For this review, take the finished solid that the model builds, in its own axes (mm). Face numbers are marked on the shaded views. A direction names the side the tool comes from. Coordinates: 2 decimals unless noted, no trailing zeros. Write each loop counter-clockwise with the first axis right and the second up, starting at its lowest first coordinate (ties: lowest second). Pieces come first, ordered by that corner, then holes. Notation, with made-up numbers: M 14,-18 L 48,-18 A11 ccw 48,3 Z; hole C 32.25,87 d7. An arc over 180 degrees is marked long. Return JSON: item names as keys, results as strings.
```python
from build123d import *

# Parameters (mm, degrees)
F0_R     = 3.8651
F1_DEPTH = 5.41
F2_R     = 2.977189
F2_R_2   = 1.369861
F3_DEPTH = 2
F4_DEPTH = 1


with BuildPart() as f1:
    # F0 (on Front) → F1 (new body)
    with BuildSketch(Plane.XZ):
        with Locations((30.719768, 18.937557)):
            Circle(F0_R)
        with BuildLine():
            ThreePointArc((28.998524, 19.481013), (29.488314, 20.257233), (30.296515, 20.692231))
            Line((30.296515, 20.692231), (30.296515, 21.202457))
            Line((30.296515, 21.202457), (31.296515, 21.202457))
            Line((31.296515, 21.202457), (31.296515, 20.647933))
            ThreePointArc((31.296515, 20.647933), (32.008417, 20.201443), (32.441011, 19.481013))
            Line((32.441011, 19.481013), (32.984868, 19.481013))
            Line((32.984868, 19.481013), (32.984868, 18.481013))
            Line((32.984868, 18.481013), (32.466076, 18.481013))
            ThreePointArc((32.466076, 18.481013), (32.039681, 17.706356), (31.296515, 17.22718))
            Line((31.296515, 17.22718), (31.296515, 16.672457))
            Line((31.296515, 16.672457), (30.296515, 16.672457))
            Line((30.296515, 16.672457), (30.296515, 17.182882))
            ThreePointArc((30.296515, 17.182882), (29.455634, 17.64915), (28.973459, 18.481013))
            Line((28.973459, 18.481013), (28.454868, 18.481013))
            Line((28.454868, 18.481013), (28.454868, 19.481013))
            Line((28.454868, 19.481013), (28.998524, 19.481013))
        make_face(mode=Mode.SUBTRACT)
    extrude(amount=F1_DEPTH)

    # F2 (on Front) → F3 (join)
    with BuildSketch(Plane.XZ):
        with Locations((30.680057, 18.935421)):
            Circle(F2_R)
        with Locations((30.680057, 18.935421)):
            Circle(F2_R_2, mode=Mode.SUBTRACT)
    extrude(amount=F3_DEPTH)

    # F2 (on Front) → F4 (cut)
    with BuildSketch(Plane.XZ):
        with Locations((30.680057, 18.935421)):
            Circle(F2_R)
        with Locations((30.680057, 18.935421)):
            Circle(F2_R_2, mode=Mode.SUBTRACT)
    extrude(amount=F4_DEPTH, mode=Mode.SUBTRACT)


solid = f1.part
```
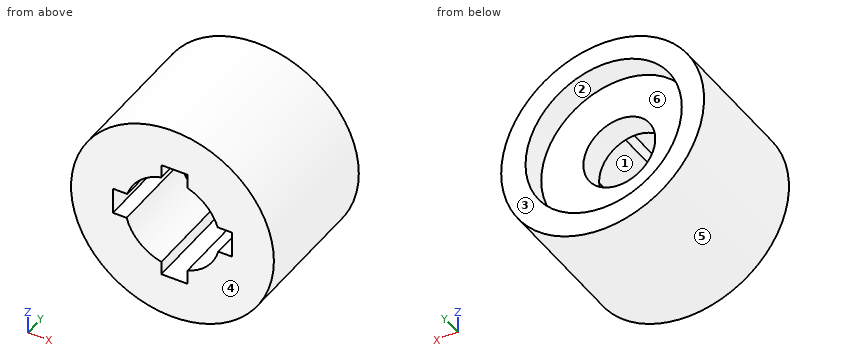
1. We need section A-A (z = 18.75). State the section outline as (x, y) points.
Checks:
{"outline": "M 26.86,-5.41 L 28.45,-5.41 L 28.45,-2 L 29.32,-2 L 29.32,-1 L 27.71,-1 L 27.71,0 L 26.86,0 Z; M 32.04,-2 L 32.98,-2 L 32.98,-5.41 L 34.58,-5.41 L 34.58,0 L 33.65,0 L 33.65,-1 L 32.04,-1 Z"}
2. Wall thickness on L1, parallel to Y at x = 29.5, z = 18; L2, parallel to Z at x = 32.5, y = -2.35; L3, parallel to Z at x = 29.75, y = -3: over which ranges is each line inside the solid? List them lowest first. Write a range as from..to.
Checks:
{"L1": "-2..-1", "L2": "15.51..18.48, 19.48..22.37", "L3": "15.2..17.42, 20.46..22.68"}
3. We need section B-B (y = -4.1). State the section outline as (x, z) points (3 decimals), plus the area to 3 significant figures.
Checks:
{"outline": "C 30.72,18.938 d7.73; hole M 28.455,18.481 L 28.973,18.481 A1.805 ccw 30.297,17.183 L 30.297,16.672 L 31.297,16.672 L 31.297,17.227 A1.805 ccw 32.466,18.481 L 32.985,18.481 L 32.985,19.481 L 32.441,19.481 A1.805 ccw 31.297,20.648 L 31.297,21.202 L 30.297,21.202 L 30.297,20.692 A1.805 ccw 28.999,19.481 L 28.455,19.481 Z", "area": "34.8 mm2"}
4. Draft analysis for pull direction Z (two halves, no side actions). For the marked faces 4, 5 and 6, state which applies: +Z half, -Z half, draft (parallel to the pull), parting line (faces both ways), or undercut.
Checks:
{"face 4": "draft", "face 5": "parting line", "face 6": "undercut"}
5. We need section C-C (x = 29.75). State the section outline as (y, z) points.
Checks:
{"outline": "M -5.41,15.2 L 0,15.2 L 0,16.11 L -1,16.11 L -1,17.93 L -2,17.93 L -2,17.42 L -5.41,17.42 Z; M -5.41,20.46 L -2,20.46 L -2,19.94 L -1,19.94 L -1,21.76 L 0,21.76 L 0,22.68 L -5.41,22.68 Z"}
6. For the marked faces 1, 2 and 3, list the 3-axis set-ups (+Z, -Z, +X, -X, +Y, -Y) from which the entire face can be reached by the end or side of a thin tool; tool diameter is ignored.
Checks:
{"face 1": "-Y", "face 2": "+Y", "face 3": "+Z, -Z, +X, -X, +Y"}
7. We need section D-D (z = 17). State the section outline as (x, y) points.
Checks:
{"outline": "M 27.38,-5.41 L 30.3,-5.41 L 30.3,-2 L 31.3,-2 L 31.3,-5.41 L 34.06,-5.41 L 34.06,0 L 32.94,0 L 32.94,-1 L 28.42,-1 L 28.42,0 L 27.38,0 Z"}
8. Clearance check with flat-ended pins moving along their axes: pin 1 Ø4 at (x, z) = (29.5, 17) entering from +Y; pin 2 Ø1.6 at (x, z) = (30.68, 18.94) entering from +Y. State where each tip first meets the part, or that it passes through.
Checks:
{"pin 1": "y = 0", "pin 2": "through"}
